Part model, mm, in its own coordinate system. A direction names the side the tool comes from. Give positions to 0.01 mm unless a question says otherwise; leave off trailing zeros. Write each loop counter-clockwise with the first axis right and the second up, starting at its lowest first coordinate (ties: lowest second). Pieces come first, ordered by that corner, then holes. Notation, with made-up numbers: M 30.25,69 L 68.25,69 A34 cw 68.25,102 Z; hole C -22.75,74.25 d11. An arc over 180 degrees is marked long. Write item = value, one per line. Start each with the question number.
from build123d import *

# Parameters (mm, degrees)
PAD009_DEPTH         = 5.4
SKETCH014_R          = 5.03
PAD010_DEPTH         = 26
PAD011_DEPTH         = 40.5
SKETCH018_R          = 1.4
POCKET005_DEPTH      = 0.001
POCKET005_DEPTH_BACK = 40.501
FILLET003_R          = 1
SKETCH031_R          = 14.133118
SKETCH031_R_2        = 9
POCKET010_DEPTH      = 40.501


with BuildPart() as part:
    # Sketch013 → Pad009 (new body, symmetric)
    with BuildSketch(Plane.XZ):
        with BuildLine():
            Line((9, 14), (9, 0))
            Line((-9, 0), (9, 0))
            Line((-9, 0), (-9, 14))
            ThreePointArc((9, 14), (0, 19.047512), (-9, 14))
        make_face()
    extrude(amount=PAD009_DEPTH, both=True)

    # Sketch014 → Pad010 (join)
    with BuildSketch(Plane.XY):
        Circle(SKETCH014_R)
    extrude(amount=PAD010_DEPTH)

    # Sketch015 → Pad011 (join)
    with BuildSketch(Plane.XY):
        Polygon((0, 4.6), (-3.983717, 2.3), (-3.983717, -2.3), (0, -4.6), (3.983717, -2.3), (3.983717, 2.3), align=None)
    extrude(amount=PAD011_DEPTH)

    # Sketch017 → Revolution002 (revolve)
    with BuildSketch(Plane.YZ):
        with BuildLine():
            Line((0, 26), (5.03, 26))
            ThreePointArc((5.03, 26), (2.706515, 27.481661), (0, 28))
            Line((0, 26), (0, 28))
        make_face()
    revolve(axis=Axis((0, 0, 0), (0, 0, 1)))

    # Sketch018 → Pocket005 (cut, two sides)
    with BuildSketch(Plane.XY) as pocket005_sk:
        Circle(SKETCH018_R)
    extrude(amount=-POCKET005_DEPTH, mode=Mode.SUBTRACT)
    extrude(pocket005_sk.sketch, amount=POCKET005_DEPTH_BACK, mode=Mode.SUBTRACT)

    # Fillet003
    fillet003_edges = [part.edges().sort_by_distance(p)[0] for p in [
        (0, 5.4, 19.047512),
        (0, -5.4, 19.047512),
        (-9, 0, 14),
        (9, 0, 14),
    ]]
    fillet(fillet003_edges, radius=FILLET003_R)

    # Sketch031 → Pocket010 (cut, through all)
    with BuildSketch(Plane.XY):
        Circle(SKETCH031_R)
        Circle(SKETCH031_R_2, mode=Mode.SUBTRACT)
    extrude(amount=POCKET010_DEPTH, mode=Mode.SUBTRACT)


solid = part.part
Q1. Tool access for faces 1 (the face through (1.96, -3.47, 33.34)), 2 (the face through (4.8, 1.5, 21.8)), 3 (the face through (-1.96, 3.47, 33.34)), 4 (the face through (-2.02, -3.434, 33.339)): list every direction of +Z, -Z, +X, -X, +Y, -Y with a clear straight run to the whole face (end or side of a thin tool).
Q2. Slice it at A-A (z = 8.5). Give the cut face in (x, y), and give its area (3 significant figures).
Q3. Probe line 1 along X through (y, z) = (0, 13.5); line 2 along Y through (x, z) = (0, 13); line 3 along Y through (x, z) = (0, 30.5). List the from-to ranges inside material, lowest first.
Q4. Two-plate mould, pull along Y, no slides. Class faces 5 (the face through (2.02, 3.434, 33.339)), 6 (the face through (-1.4, 0.06, 19.97)), 7 (the face through (-3.984, 0, 33)): +Y half, -Y half, draft (parallel to the pull), parting line (faces both ways), or undercut.
Q5. Slice it at B-B (z = 23). Give the cut face in (x, y).
Q6. Drop flat-ended pins along their axis: P1, Ø1, axis at y = 1, z = 12.5, coming from the +X side; P2, Ø3, axis at y = 2, z = 4, coming from the -X side; P3, Ø2.5, axis at x = 0, y = 0, coming from the +Z side; P4, Ø8, axis at x = 6.5, z = 30, coming from the +Y side. Give the stop position or say it passes through.
Working result:
q1.face_1 = +Z, +X, -Y
q1.face_2 = +Z
q1.face_3 = +Z, -X, +Y
q1.face_4 = +Z, -X, -Y
q2.outline = M -7.2,-5.4 L 7.2,-5.4 A9 ccw 7.2,5.4 L -7.2,5.4 A9 ccw Z; hole C 0,0 d2.8
q2.area = 176 mm2
q3.line_1 = -9 to -1.4, 1.4 to 9
q3.line_2 = -5.4 to -1.4, 1.4 to 5.4
q3.line_3 = -4.6 to -1.4, 1.4 to 4.6
q4.face_5 = +Y half
q4.face_6 = undercut
q4.face_7 = draft
q5.outline = C 0,0 d10.06; hole C 0,0 d2.8
q6.P1 = 8.99
q6.P2 = -8.99
q6.P3 = through
q6.P4 = 3.16
